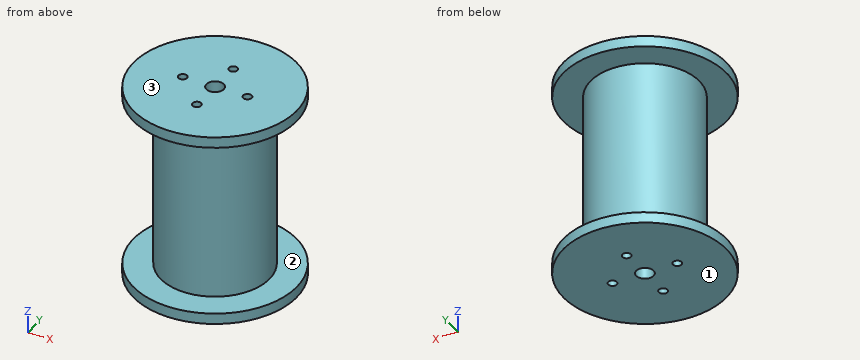
```python
from build123d import *

# Parameters (mm, degrees)
SKETCH1_R           = 25
BOSS_EXTRUDE1_DEPTH = 80
SKETCH2_R           = 37.5
BOSS_EXTRUDE2_DEPTH = 5
BOSS_EXTRUDE3_START = 5
SKETCH3_R           = 37.5
BOSS_EXTRUDE3_DEPTH = 5
SKETCH4_R           = 4
SKETCH4_R_2         = 2
CUT_EXTRUDE1_DEPTH  = 105.462912079


with BuildPart() as part:
    # Sketch1 → Boss-Extrude1 (new body)
    with BuildSketch(Plane.XY):
        Circle(SKETCH1_R)
    extrude(amount=BOSS_EXTRUDE1_DEPTH)

    # Sketch2 → Boss-Extrude2 (add)
    with BuildSketch(Plane.XY.offset(80)):
        Circle(SKETCH2_R)
    extrude(amount=BOSS_EXTRUDE2_DEPTH)

    # Sketch3 → Boss-Extrude3 (add)
    with BuildSketch(Plane(origin=(0, 0, 0), x_dir=(-1, 0, 0), z_dir=(0, 0, -1)).offset(BOSS_EXTRUDE3_START)):
        with Locations(Location((0, 0, 0), (0, 0, 180))):
            Circle(SKETCH3_R)
    extrude(amount=-BOSS_EXTRUDE3_DEPTH)

    # Sketch4 → Cut-Extrude1 (cut, through all)
    with BuildSketch(Plane(origin=(0, 0, -5), x_dir=(-1, 0, 0), z_dir=(0, 0, -1))):
        Circle(SKETCH4_R)
        with Locations((0, 15)):
            Circle(SKETCH4_R_2)
        with Locations((15, 0)):
            Circle(SKETCH4_R_2)
        with Locations((0, -15)):
            Circle(SKETCH4_R_2)
        with Locations((-15, 0)):
            Circle(SKETCH4_R_2)
    extrude(amount=-CUT_EXTRUDE1_DEPTH, mode=Mode.SUBTRACT)


solid = part.part
```
Work out the finished part from the listing and answer in its coordinate system (mm). Face numbers are marked on the shaded views. Round coordinates to 2 decimals unless told otherwise and drop trailing zeros. Loops run counter-clockwise (first coordinate to the right, second up) from the corner with the lowest first, then second, coordinate; pieces in that order, holes last.
(1) The part is cut by section B-B, the plane z = 77.5. Give the vertices of the cut face in (x, y), and give its area (3 significant figures).
Computed values:
outline: circle Ø50 at (0, 0); hole circle Ø4 at (-15, 0); hole circle Ø8 at (0, 0); hole circle Ø4 at (0, -15); hole circle Ø4 at (0, 15); hole circle Ø4 at (15, 0)
area: 1,860 mm2
(2) Each of these flat-tipped pins is pushed along its axis until it touches: P1, Ø1, axis at x = -10.5, z = 53.5, coming from the -Y side; P2, Ø3, axis at y = -18.5, z = 6.5, coming from the -X side; P3, Ø12, axis at x = -14.5, z = 56, coming from the +Y side. Where does it stop, or does it pass through?
Computed values:
P1: stops at y = -22.91
P2: stops at x = -18.33
P3: stops at y = 23.51
(3) The part is cut by section D-D, the plane x = 0. Give the vertices of the cut face in (y, z).
Computed values:
outline: (-37.5, -5) - (-17, -5) - (-17, 85) - (-37.5, 85) - (-37.5, 80) - (-25, 80) - (-25, 0) - (-37.5, 0) - close; (-13, -5) - (-4, -5) - (-4, 85) - (-13, 85) - close; (4, -5) - (13, -5) - (13, 85) - (4, 85) - close; (17, -5) - (37.5, -5) - (37.5, 0) - (25, 0) - (25, 80) - (37.5, 80) - (37.5, 85) - (17, 85) - close
(4) The mould has two halves that part along Z. Classify the marked faces 1, 2 and 3: pulls with the +Z half, pulls with the -Z half, needs draft (parallel to the pull), parting line crosses it, or undercut.
Computed values:
face 1: pulls with the -Z half
face 2: undercut
face 3: pulls with the +Z half
(5) Find the intervals of material crossed by L1, parallel to Z at x = -17, y = 33; L2, parallel to X at y = 1, z = 41.5; L3, parallel to Y at x = -15, z = 63.5, in increasing order.
Computed values:
L1: z = -5 to 0, 80 to 85
L2: x = -24.98 to -16.73, -13.27 to -3.87, 3.87 to 13.27, 16.73 to 24.98
L3: y = -20 to -2, 2 to 20
(6) The part is cut by section C-C, the plane y = 30.5. Give the vertices of the cut face in (x, z).
Computed values:
outline: (-21.82, -5) - (21.82, -5) - (21.82, 0) - (-21.82, 0) - close; (-21.82, 80) - (21.82, 80) - (21.82, 85) - (-21.82, 85) - close
(7) The part is cut by section A-A, the plane x = 30. Give the vertices of the cut face in (y, z).
Computed values:
outline: (-22.5, -5) - (22.5, -5) - (22.5, 0) - (-22.5, 0) - close; (-22.5, 80) - (22.5, 80) - (22.5, 85) - (-22.5, 85) - close
